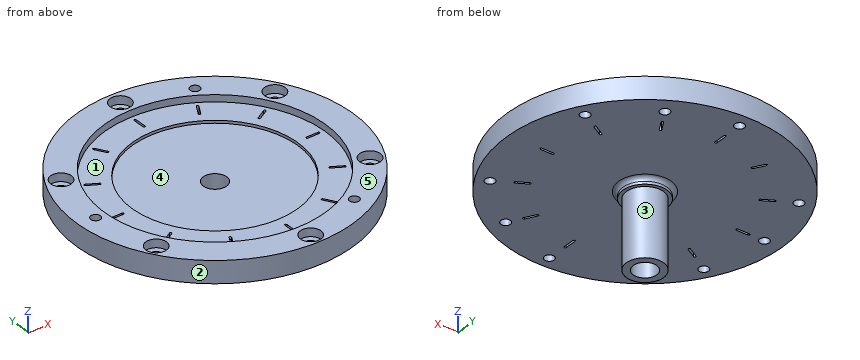
from build123d import *

# Parameters (mm, degrees)
SKETCH2_R                               = 200
BOSS_EXTRUDE1_DEPTH                     = 32
CBORE_FOR_M5_HEX_HEAD_BOLT2_D           = 14
CBORE_FOR_M5_HEX_HEAD_BOLT2_CBORE_D     = 30
CBORE_FOR_M5_HEX_HEAD_BOLT2_CBORE_DEPTH = 12
CIRPATTERN1_COUNT                       = 6
SKETCH9_R                               = 7
CUT_EXTRUDE1_DEPTH                      = 285.647149995
SKETCH12_R                              = 160
CUT_EXTRUDE7_DEPTH                      = 10
SKETCH13_R                              = 120
CUT_EXTRUDE8_DEPTH                      = 4
CUT_EXTRUDE9_DEPTH                      = 285.647149995
SKETCH16_R                              = 135
CUT_EXTRUDE10_DEPTH                     = 4
SKETCH17_R                              = 32
BOSS_EXTRUDE2_DEPTH                     = 10
FILLET1_R                               = 6
SKETCH18_R                              = 27
BOSS_EXTRUDE3_DEPTH                     = 98
SKETCH20_R                              = 21
BOSS_EXTRUDE4_DEPTH                     = 32
SKETCH19_R                              = 17
CUT_EXTRUDE11_DEPTH                     = 128


with BuildPart() as part:
    # Sketch2 → Boss-Extrude1 (new body)
    with BuildSketch(Plane.XY):
        Circle(SKETCH2_R)
    extrude(amount=BOSS_EXTRUDE1_DEPTH)

    # CBORE for M5 Hex Head Bolt2 (through all)
    with Locations(Plane.XY.offset(32)):
        with Locations((0, 180)):
            cbore_for_m5_hex_head_bolt2 = CounterBoreHole(CBORE_FOR_M5_HEX_HEAD_BOLT2_D / 2, CBORE_FOR_M5_HEX_HEAD_BOLT2_CBORE_D / 2, CBORE_FOR_M5_HEX_HEAD_BOLT2_CBORE_DEPTH)

    # CirPattern1: CBORE for M5 Hex Head Bolt2 ×6 about axis
    cirpattern1_axis = Axis((0, -1.01822753, 0), (0, 0, 1))
    for i in range(1, CIRPATTERN1_COUNT):
        add(cbore_for_m5_hex_head_bolt2.rotate(cirpattern1_axis, i * 360 / CIRPATTERN1_COUNT), mode=Mode.SUBTRACT)

    # Sketch9 → Cut-Extrude1 (cut, through all)
    with BuildSketch(Plane.XY.offset(32)):
        with Locations((-175, 0)):
            Circle(SKETCH9_R)
        with Locations((87.5, 151.554445662)):
            Circle(SKETCH9_R)
        with Locations((87.5, -151.554445662)):
            Circle(SKETCH9_R)
    extrude(amount=-CUT_EXTRUDE1_DEPTH, mode=Mode.SUBTRACT)

    # Sketch12 → Cut-Extrude7 (cut)
    with BuildSketch(Plane.XY.offset(32)):
        Circle(SKETCH12_R)
    extrude(amount=-CUT_EXTRUDE7_DEPTH, mode=Mode.SUBTRACT)

    # Sketch13 → Cut-Extrude8 (cut)
    with BuildSketch(Plane.XY.offset(22)):
        Circle(SKETCH13_R)
    extrude(amount=-CUT_EXTRUDE8_DEPTH, mode=Mode.SUBTRACT)

    # Sketch15 → Cut-Extrude9 (cut, through all)
    with BuildSketch(Plane(origin=(0, 0, 0), x_dir=(-1, 0, 0), z_dir=(0, 0, -1))):
        with BuildLine():
            Line((1.5, -135), (1.5, -152.035767594))
            ThreePointArc((1.5, -152.035767594), (0, -153.535767594), (-1.5, -152.035767594))
            Line((-1.5, -152.035767594), (-1.5, -135))
            ThreePointArc((-1.5, -135), (0, -133.5), (1.5, -135))
        make_face()
        with BuildLine():
            Line((-66.200961894, -117.663429511), (-74.718845691, -132.41683702))
            ThreePointArc((-74.718845691, -132.41683702), (-76.767883797, -132.965875126), (-77.316921902, -130.91683702))
            Line((-77.316921902, -130.91683702), (-68.799038106, -116.163429511))
            ThreePointArc((-68.799038106, -116.163429511), (-66.75, -115.614391405), (-66.200961894, -117.663429511))
        make_face()
        with BuildLine():
            Line((-116.163429511, -68.799038106), (-130.91683702, -77.316921902))
            ThreePointArc((-130.91683702, -77.316921902), (-132.965875126, -76.767883797), (-132.41683702, -74.718845691))
            Line((-132.41683702, -74.718845691), (-117.663429511, -66.200961894))
            ThreePointArc((-117.663429511, -66.200961894), (-115.614391405, -66.75), (-116.163429511, -68.799038106))
        make_face()
        with BuildLine():
            Line((-135, -1.5), (-152.035767594, -1.5))
            ThreePointArc((-152.035767594, -1.5), (-153.535767594, 0), (-152.035767594, 1.5))
            Line((-152.035767594, 1.5), (-135, 1.5))
            ThreePointArc((-135, 1.5), (-133.5, 0), (-135, -1.5))
        make_face()
        with BuildLine():
            Line((-117.663429511, 66.200961894), (-132.41683702, 74.718845691))
            ThreePointArc((-132.41683702, 74.718845691), (-132.965875126, 76.767883797), (-130.91683702, 77.316921902))
            Line((-130.91683702, 77.316921902), (-116.163429511, 68.799038106))
            ThreePointArc((-116.163429511, 68.799038106), (-115.614391405, 66.75), (-117.663429511, 66.200961894))
        make_face()
        with BuildLine():
            Line((-68.799038106, 116.163429511), (-77.316921902, 130.91683702))
            ThreePointArc((-77.316921902, 130.91683702), (-76.767883797, 132.965875126), (-74.718845691, 132.41683702))
            Line((-74.718845691, 132.41683702), (-66.200961894, 117.663429511))
            ThreePointArc((-66.200961894, 117.663429511), (-66.75, 115.614391405), (-68.799038106, 116.163429511))
        make_face()
        with BuildLine():
            Line((-1.5, 135), (-1.5, 152.035767594))
            ThreePointArc((-1.5, 152.035767594), (0, 153.535767594), (1.5, 152.035767594))
            Line((1.5, 152.035767594), (1.5, 135))
            ThreePointArc((1.5, 135), (0, 133.5), (-1.5, 135))
        make_face()
        with BuildLine():
            Line((66.200961894, 117.663429511), (74.718845691, 132.41683702))
            ThreePointArc((74.718845691, 132.41683702), (76.767883797, 132.965875126), (77.316921902, 130.91683702))
            Line((77.316921902, 130.91683702), (68.799038106, 116.163429511))
            ThreePointArc((68.799038106, 116.163429511), (66.75, 115.614391405), (66.200961894, 117.663429511))
        make_face()
        with BuildLine():
            Line((116.163429511, 68.799038106), (130.91683702, 77.316921902))
            ThreePointArc((130.91683702, 77.316921902), (132.965875126, 76.767883797), (132.41683702, 74.718845691))
            Line((132.41683702, 74.718845691), (117.663429511, 66.200961894))
            ThreePointArc((117.663429511, 66.200961894), (115.614391405, 66.75), (116.163429511, 68.799038106))
        make_face()
        with BuildLine():
            Line((135, 1.5), (152.035767594, 1.5))
            ThreePointArc((152.035767594, 1.5), (153.535767594, 0), (152.035767594, -1.5))
            Line((152.035767594, -1.5), (135, -1.5))
            ThreePointArc((135, -1.5), (133.5, 0), (135, 1.5))
        make_face()
        with BuildLine():
            Line((117.663429511, -66.200961894), (132.41683702, -74.718845691))
            ThreePointArc((132.41683702, -74.718845691), (132.965875126, -76.767883797), (130.91683702, -77.316921902))
            Line((130.91683702, -77.316921902), (116.163429511, -68.799038106))
            ThreePointArc((116.163429511, -68.799038106), (115.614391405, -66.75), (117.663429511, -66.200961894))
        make_face()
        with BuildLine():
            Line((68.799038106, -116.163429511), (77.316921902, -130.91683702))
            ThreePointArc((77.316921902, -130.91683702), (76.767883797, -132.965875126), (74.718845691, -132.41683702))
            Line((74.718845691, -132.41683702), (66.200961894, -117.663429511))
            ThreePointArc((66.200961894, -117.663429511), (66.75, -115.614391405), (68.799038106, -116.163429511))
        make_face()
    extrude(amount=-CUT_EXTRUDE9_DEPTH, mode=Mode.SUBTRACT)

    # Sketch16 → Cut-Extrude10 (cut)
    with BuildSketch(Plane.XY.offset(18)):
        Circle(SKETCH16_R)
    extrude(amount=-CUT_EXTRUDE10_DEPTH, mode=Mode.SUBTRACT)

    # Sketch17 → Boss-Extrude2 (add)
    with BuildSketch(Plane(origin=(0, 0, 0), x_dir=(-1, 0, 0), z_dir=(0, 0, -1))):
        with Locations(Location((0, 0, 0), (0, 0, 180))):
            Circle(SKETCH17_R)
    extrude(amount=BOSS_EXTRUDE2_DEPTH)

    # Fillet1
    fillet1_edges = [part.edges().sort_by_distance(p)[0] for p in [
        (-32, 0, 0),
    ]]
    fillet(fillet1_edges, radius=FILLET1_R)

    # Sketch18 → Boss-Extrude3 (add)
    with BuildSketch(Plane(origin=(0, 0, -10), x_dir=(-1, 0, 0), z_dir=(0, 0, -1))):
        Circle(SKETCH18_R)
    extrude(amount=BOSS_EXTRUDE3_DEPTH)

    # Sketch20 → Boss-Extrude4 (add)
    with BuildSketch(Plane(origin=(0, 0, -108), x_dir=(-1, 0, 0), z_dir=(0, 0, -1))):
        Circle(SKETCH20_R)
    extrude(amount=-BOSS_EXTRUDE4_DEPTH)

    # Sketch19 → Cut-Extrude11 (cut)
    with BuildSketch(Plane(origin=(0, 0, -108), x_dir=(-1, 0, 0), z_dir=(0, 0, -1))):
        Circle(SKETCH19_R)
    extrude(amount=-CUT_EXTRUDE11_DEPTH, mode=Mode.SUBTRACT)


solid = part.part
Read the model definition and answer for the solid it produces. Units are mm, in the model's axes. Face numbers are marked on the shaded views. A direction names the side the tool comes from. Coordinates: 2 decimals unless noted, no trailing zeros. Write each loop counter-clockwise with the first axis right and the second up, starting at its lowest first coordinate (ties: lowest second). Pieces come first, ordered by that corner, then holes. Notation, with made-up numbers: (49, -13) -> (60, -13) arc R24 cw to (60, 17) -> close; hole circle Ø5 at (-39.5, 18.5). An arc over 180 degrees is marked (long way). Return JSON: item names as keys, results as strings.
(1) The part is cut by section B-B on z = -76.5. Give the vertices of the cut face in (x, y).
Answers below:
{"outline": "circle Ø54 at (0, 0); hole circle Ø34 at (0, 0)"}
(2) For a pull along Y with two mould halves and no side action, classify the marked faces 3, 4 and 5 as pulls with the +Y half, pulls with the -Y half, needs draft (parallel to the pull), parting line crosses it, or undercut.
Answers below:
{"face 3": "parting line crosses it", "face 4": "undercut", "face 5": "needs draft"}
(3) The part is cut by section C-C on x = 88. Give the vertices of the cut face in (y, z).
Answers below:
{"outline": "(-179.6, 0) -> (-158.54, 0) -> (-158.54, 32) -> (-179.6, 32) -> close; (-144.57, 0) -> (144.57, 0) -> (144.57, 32) -> (133.63, 32) -> (133.63, 22) -> (81.58, 22) -> (81.58, 18) -> (102.38, 18) -> (102.38, 14) -> (-102.38, 14) -> (-102.38, 18) -> (-81.58, 18) -> (-81.58, 22) -> (-133.63, 22) -> (-133.63, 32) -> (-144.57, 32) -> close; (158.54, 0) -> (179.6, 0) -> (179.6, 32) -> (158.54, 32) -> close"}
(4) The part is cut by section A-A on y = 180. Give the vertices of the cut face in (x, z).
Answers below:
{"outline": "(-87.18, 0) -> (-7, 0) -> (-7, 20) -> (-15, 20) -> (-15, 32) -> (-87.18, 32) -> close; (7, 0) -> (87.18, 0) -> (87.18, 32) -> (15, 32) -> (15, 20) -> (7, 20) -> close"}
(5) Which of the six approach directions +Z, -Z, +X, -X, +Y, -Y give full straight-line access (tool end or side, diameter ignored) to the marked faces 1 and 2?
Answers below:
{"face 1": "+Z", "face 2": "+Z, -Z"}
(6) Consider line 1 along Y through (x, z) = (69.5, 9.5); line 2 along Y through (x, z) = (0, -62); line 3 along Z through (x, y) = (158, 13). Determine where each line is inside the solid, lowest interval first. Write a range as from..to.
Answers below:
{"line 1": "-187.54..-123.38, -117.38..117.38, 123.38..187.54", "line 2": "-27..-17, 17..27", "line 3": "0..22"}
(7) Each of these flat-tipped pins is pushed along its axis until it touches: P1, Ø6, axis at x = -17.5, z = 6, coming from the +Y side; P2, Ø15, axis at x = 5, y = -185.5, coming from the +Z side; P3, Ø4, axis at y = -6.5, z = -36.5, coming from the -X side. Where does it stop, or does it pass through?
Answers below:
{"P1": "y = 199.47", "P2": "z = 20", "P3": "x = -26.62"}
